Design review of the part shown in the three views and the two pictorial views. Dimensions are in mm from the part's minimum x, y and z. A direction names the side the tool comes from. Coordinates: 2 decimals unless noted, no trailing zeros. Order: outer loops, then holes, each group sorted by start corner. A loop starts at its lowest first (then second) coordinate and runs counter-clockwise, first axis right, second up. Notation, with made-up numbers: (36, -23) -> (95, -23) arc R20 ccw to (95, -15) -> close; hole circle Ø5 at (83, 78). An arc over 180 degrees is marked (long way). Answer as a JSON object with one key per item and string values. Group by question number.
1) For pin 1 (1 mm diameter, centred on x = 23.5, z = 0.5, fed in from -Y); pin 2 (1.8 mm diameter, centred on y = 12.5, z = 2, fed in from +X), all flat-tipped, find the tip position at first contact; note any pin that passes through.
2) Draft analysis for pull direction Y (two halves, no side actions). For the marked faces 1, 2 and 3, state which applies: +Y half, -Y half, draft (parallel to the pull), parting line (faces both ways), or undercut.
3) Add section B-B, the plane x = 7.5. Write out the cut boundary in (y, z).
4) Add section D-D, the plane x = 25. Write out the cut boundary in (y, z), then the cut area to 3 significant figures.
5) Machinability: for the marked faces 4 and 5, which of the approach directions +Z, -Z, +X, -X, +Y, -Y give a long, thin tool a straight path to every point of the face, cutting with its end or side? Answer none if there is none.
6) Add section C-C, the plane z = 1.2. Write out the cut boundary in (x, y).
7) Add section A-A, the plane y = 32.5. Write out the cut boundary in (x, z).
8) Wall thickness on L1, parallel to Y at x = 7.5, z = 3.25; L2, parallel to Y at x = 7.5, z = 1.3; L3, parallel to X at y = 23, z = 3: over which ranges is each line inside the solid? List them lowest first.
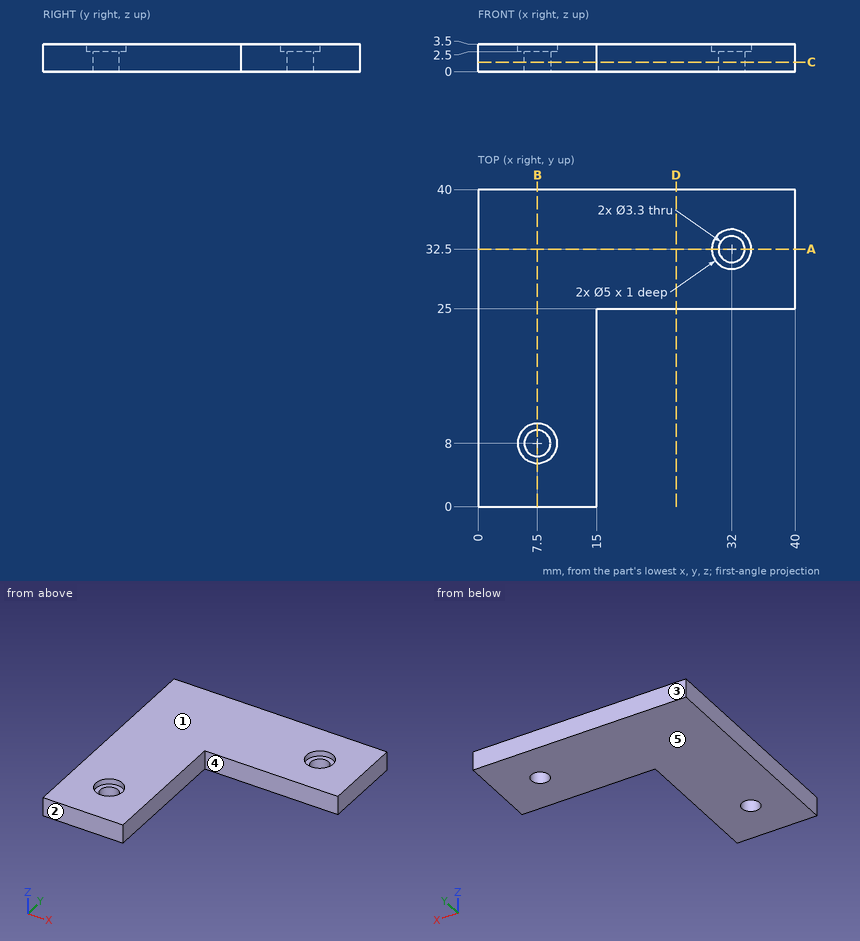
Output values:
{
 "1": {"pin 1": "stops at y = 25", "pin 2": "stops at x = 15"},
 "2": {"face 1": "draft", "face 2": "-Y half", "face 3": "+Y half"},
 "3": {"outline": "(0, 0) -> (6.35, 0) -> (6.35, 2.5) -> (5.5, 2.5) -> (5.5, 3.5) -> (0, 3.5) -> close; (9.65, 0) -> (40, 0) -> (40, 3.5) -> (10.5, 3.5) -> (10.5, 2.5) -> (9.65, 2.5) -> close"},
 "4": {"outline": "(25, 0) -> (40, 0) -> (40, 3.5) -> (25, 3.5) -> close", "area": "52.5 mm²"},
 "5": {"face 4": "+Z, -Z, +X, -Y", "face 5": "-Z, +X, -X, +Y, -Y"},
 "6": {"outline": "(0, 0) -> (15, 0) -> (15, 25) -> (40, 25) -> (40, 40) -> (0, 40) -> close; hole circle Ø3.3 at (7.5, 8); hole circle Ø3.3 at (32, 32.5)"},
 "7": {"outline": "(0, 0) -> (30.35, 0) -> (30.35, 2.5) -> (29.5, 2.5) -> (29.5, 3.5) -> (0, 3.5) -> close; (33.65, 0) -> (40, 0) -> (40, 3.5) -> (34.5, 3.5) -> (34.5, 2.5) -> (33.65, 2.5) -> close"},
 "8": {"L1": "y = 0 to 5.5, 10.5 to 40", "L2": "y = 0 to 6.35, 9.65 to 40", "L3": "x = 0 to 15"}
}
